from build123d import *

# Parameters (mm, degrees)
BASE_FLANGE1_DEPTH = 10
CUT_EXTRUDE1_DEPTH = 2.032
CUT_EXTRUDE2_DEPTH = 2.032


# Sheet-metal steps are written as plain solids
with BuildPart() as part:
    # Sketch1 → Base-Flange1 (new, symmetric)
    with BuildSketch(Plane.XY):
        with BuildLine():
            Line((-17.225320151, -6), (-0.707106781, 10.51821337))
            ThreePointArc((-0.707106781, 10.51821337), (0, 10.811106589), (0.707106781, 10.51821337))
            Line((0.707106781, 10.51821337), (15.081372391, -3.856052239))
            ThreePointArc((15.081372391, -3.856052239), (17.225320151, -4.744104479), (19.369267912, -3.856052239))
            Line((19.369267912, -3.856052239), (85.932426933, 62.707106781))
            ThreePointArc((85.932426933, 62.707106781), (86.256850281, 62.923879533), (86.639533714, 63))
            Line((86.639533714, 63), (135, 63))
            Line((135, 63), (135, 65.032))
            Line((135, 65.032), (86.639533714, 65.032))
            ThreePointArc((86.639533714, 65.032), (85.479237547, 64.801202743), (84.495585953, 64.143947761))
            Line((84.495585953, 64.143947761), (17.932426933, -2.41921126))
            ThreePointArc((17.932426933, -2.41921126), (17.225320151, -2.712104479), (16.51821337, -2.41921126))
            Line((16.51821337, -2.41921126), (2.143947761, 11.95505435))
            ThreePointArc((2.143947761, 11.95505435), (0, 12.843106589), (-2.143947761, 11.95505435))
            Line((-2.143947761, 11.95505435), (-18.662161131, -4.563159021))
            Line((-18.662161131, -4.563159021), (-17.225320151, -6))
        make_face()
    extrude(amount=BASE_FLANGE1_DEPTH, both=True)

    # Sketch6 → Cut-Extrude1 (cut)
    with BuildSketch(Plane(origin=(-7.049501055, 7.049501055, 0), x_dir=(0, 0, 1), z_dir=(-0.7071067811865488, 0.7071067811865464, 0))):
        with BuildLine():
            Line((-5, -5), (5, -5))
            ThreePointArc((5, -5), (8, -8), (5, -11))
            Line((5, -11), (-5, -11))
            ThreePointArc((-5, -11), (-8, -8), (-5, -5))
        make_face()
    extrude(amount=-CUT_EXTRUDE1_DEPTH, mode=Mode.SUBTRACT)

    # Sketch9 → Cut-Extrude2 (cut)
    with BuildSketch(Plane(origin=(7.049501055, 7.049501055, 0), x_dir=(0, 0, -1), z_dir=(0.7071067811865488, 0.7071067811865464, 0))):
        with BuildLine():
            Line((-5, -3), (5, -3))
            ThreePointArc((5, -3), (8, -6), (5, -9))
            Line((5, -9), (-5, -9))
            ThreePointArc((-5, -9), (-8, -6), (-5, -3))
        make_face()
    extrude(amount=-CUT_EXTRUDE2_DEPTH, mode=Mode.SUBTRACT)


solid = part.part
The model under review builds one solid part; all positions refer to its coordinate system, in mm. A direction names the side the tool comes from. Round coordinates to 2 decimals unless told otherwise and drop trailing zeros. Loops run counter-clockwise (first coordinate to the right, second up) from the corner with the lowest first, then second, coordinate; pieces in that order, holes last. Notation, with made-up numbers: (36, 31) -> (72, 31) arc R15 cw to (72, 48) -> close; hole circle Ø4 at (28, 17). An arc over 180 degrees is marked (long way). Write item = value, one per line. Start each with the question number.
Item 1: Take a section at D-D on z = -6.5. Give the boundary of the cut face in (x, y), plus the area to 3 significant figures.
Item 2: For faces 4 (the cylindrical face through (-12, 0.7, 8)), 5 (the flat face through (6.196, 5.029, 0.14)), 6 (the flat face through (111, 65.032, 0)), 7 (the flat face through (110, 63, 0)), 8 (the flat face through (51.68, 31.33, 0.14)), list the 3-axis set-ups (+Z, -Z, +X, -X, +Y, -Y) from which the entire face can be reached by the end or side of a thin tool; tool diameter is ignored.
Item 3: Insertion check: pin 1 (6 mm diameter, centred on y = 51.5, z = -2.5, fed in from -X); pin 2 (12 mm diameter, centred on y = 24.5, z = -0.5, fed in from -X); pin 3 (6 mm diameter, centred on x = 29.5, z = 7, fed in from +Y). Each pin has a flat end and moves straight along its axis. Give the tip position at first contact, or say it passes through.
Item 4: Mouldability with a two-part tool opening along Z and no side actions: class faces 1 (the cylindrical face through (10.5, 2.1, -8)), 2 (the flat face through (7.8, 6.3, 0.1)), 3 (the flat face through (58, 35, -10)) as released by +Z, released by -Z, zero draft, split by the parting line, or undercut.
Item 5: To check wall thickness, follow L1, parallel to Y at x = 109, z = 6.5; L2, parallel to X at y = 10, z = 8; L3, parallel to X at y = 12, z = -1. State the ranges of each line that lie inside material, in increasing order.
Item 6: Take a section at C-C on y = 40.5. Give the boundary of the cut face in (x, z).
Item 7: Take a section at B-B on x = 89. Give the boundary of the cut face in (y, z).
Item 8: Take a section at A-A on z = 3.5. Give the boundary of the cut face in (x, y), plus the area to 3 significant figures.
Result:
q1.outline = (-18.66, -4.56) -> (-17.23, -6) -> (-13.11, -1.88) -> (-14.54, -0.44) -> close; (-10.87, 3.23) -> (-9.43, 1.79) -> (-0.71, 10.52) arc R1 cw to (0.71, 10.52) -> (8.02, 3.21) -> (9.46, 4.64) -> (2.14, 11.96) arc R3.03 ccw to (-2.14, 11.96) -> close; (11.69, -0.47) -> (15.08, -3.86) arc R3.03 ccw to (19.37, -3.86) -> (85.93, 62.71) arc R1 cw to (86.64, 63) -> (135, 63) -> (135, 65.03) -> (86.64, 65.03) arc R3.03 ccw to (84.5, 64.14) -> (17.93, -2.42) arc R1 cw to (16.52, -2.42) -> (13.13, 0.97) -> close
q1.area = 373 mm²
q2.face_4 = none
q2.face_5 = +Z, -Z, -Y
q2.face_6 = +Z, -Z, +X, -X, +Y
q2.face_7 = +Z, -Z, +X, -Y
q2.face_8 = +Z, -Z, +Y
q3.pin_1 = 68.85
q3.pin_2 = 38.85
q3.pin_3 = 12.15
q4.face_1 = undercut
q4.face_2 = zero draft
q4.face_3 = released by -Z
q5.L1 = 63 to 65.03
q5.L2 = -4.1 to -1.23, 1.23 to 4.1, 30.35 to 33.23
q5.L3 = -2.1 to 2.1, 32.35 to 35.23
q6.outline = (60.85, -10) -> (63.73, -10) -> (63.73, 10) -> (60.85, 10) -> close
q7.outline = (63, -10) -> (65.03, -10) -> (65.03, 10) -> (63, 10) -> close
q8.outline = (-18.66, -4.56) -> (-17.23, -6) -> (-13.39, -2.17) -> (-14.83, -0.73) -> close; (-10.59, 3.51) -> (-9.15, 2.08) -> (-0.71, 10.52) arc R1 cw to (0.71, 10.52) -> (7.73, 3.49) -> (9.17, 4.93) -> (2.14, 11.96) arc R3.03 ccw to (-2.14, 11.96) -> close; (11.98, -0.75) -> (15.08, -3.86) arc R3.03 ccw to (19.37, -3.86) -> (85.93, 62.71) arc R1 cw to (86.64, 63) -> (135, 63) -> (135, 65.03) -> (86.64, 65.03) arc R3.03 ccw to (84.5, 64.14) -> (17.93, -2.42) arc R1 cw to (16.52, -2.42) -> (13.41, 0.69) -> close
q8.area = 370 mm²
